Work out the finished part from the listing and answer in its coordinate system (mm). A direction names the side the tool comes from. Give positions to 0.01 mm unless a question says otherwise; leave off trailing zeros. Loops run counter-clockwise (first coordinate to the right, second up) from the corner with the lowest first, then second, coordinate; pieces in that order, holes last.
Autodesk Fusion 360 part; units mm, degrees
sketch "Sketch1" plane through (0, 0, 0) normal (0, 1, 0) x (1, 0, 0)
  circle A0 centre (0, 0) radius 4
  circle A1 centre (0, 0) radius 25
  line L0 (0, 0) -> (-25, 0)
  line L1 (0, 0) -> (25, 0)
  line L2 (-25, 0) -> (25, 0)
  line L3 (25, 0) -> (25, 51.781)
  line L4 (25, 51.781) -> (-25, 51.781)
  line L5 (-25, 51.781) -> (-25, 0)
  line L6 (-14.5, 51.781) -> (-7.5, 51.781)
  line L7 (-7.5, 51.781) -> (-7.5, 26.781)
  line L8 (-7.5, 26.781) -> (-14.5, 26.781)
  line L9 (-14.5, 26.781) -> (-14.5, 51.781)
  line L10 (-17.5, 35.781) -> (-4.5, 35.781)
  line L11 (-4.5, 35.781) -> (-4.5, 42.781)
  line L12 (-4.5, 42.781) -> (-17.5, 42.781)
  line L13 (-17.5, 42.781) -> (-17.5, 35.781)
  line L14 (-11, 35.781) -> (-11, 26.781)
  line L15 (-17.5, 39.281) -> (-14.5, 39.281)
  line L16 (0, 51.781) -> (0, 83.1045)
  line L17 (7.5, 51.781) -> (7.5, 26.781)
  line L18 (7.5, 26.781) -> (14.5, 26.781)
  line L19 (14.5, 26.781) -> (14.5, 51.781)
  line L20 (17.5, 35.781) -> (4.5, 35.781)
  line L21 (17.5, 42.781) -> (17.5, 35.781)
  line L22 (4.5, 42.781) -> (17.5, 42.781)
  line L23 (4.5, 35.781) -> (4.5, 42.781)
  dimension "d1" = 8
  dimension "d2" = 50
  dimension "d3" = 25
  dimension "d4" = 7
  dimension "d5" = 7
  dimension "d6" = 13
  dimension "d7" = 90
  dimension "d8" = 90
  dimension "d9" = 9
  dimension "d10" = 51.781
extrude "Extrude1" add sketch "Sketch1" along normal blind 10 contours A0 A1 L0 L1 L2 | A0 A1 L0 L1 L2 | A1 L3 L4 L5 L7 L8 L9 L10 L11 L12 L13 L17 L18 L19 L20 L21 L22 L23
extrude "Extrude2" add 1 faces at (14.2683, 0, -9.6781) along direction (0, -1, 0) blind 1
Item 1: Find section D-D, the plane z = 2. Write down the section's boundary in (x, y).
Item 2: Find section B-B, the plane z = -41. Write down the section's boundary in (x, y), plus the area to 3 significant figures.
Item 3: Consider line 1 (X direction, y = 8.25, z = -42); line 2 (X direction, y = 3, z = 0); line 3 (Z direction, x = 0, y = 7.25). Determine where each line is inside the solid, lowest interval first.
Item 4: For faces 5 (the face through (25, 5, -26)), 6 (the face through (-4.5, 5, -39)), 7 (the face through (7.5, 5, -47)), determine the directions among +Z, -Z, +X, -X, +Y, -Y from which every point of the face is accessible in a straight line to the end or side of a thin tool.
Item 5: Find section A-A, the plane x = 0. Write down the section's boundary in (y, z), plus the area to 3 significant figures.
Item 6: Determine the mould class of faces 1 (the face through (14.5, 5, -47)), 2 (the face through (-6, 5, -35.781)), 3 (the face through (-20, 5, -51.781)), 4 (the face through (-16, 5, -35.781)) for opening direction Z: released by +Z, released by -Z, zero draft, split by the parting line, or undercut.
Item 7: Flat-ended cylindrical pins translate along their axes: pin 1 Ø6.5 at (x, z) = (0, 0) entering from +Y; pin 2 Ø3 at (x, y) = (15.5, 9) entering from +Z; pin 3 Ø1 at (x, y) = (-16.5, 8) entering from +Z; pin 4 Ø2.5 at (x, y) = (-16, 2.5) entering from +Z. Find the tip coordinate at first contact, or state that the pin passes through.
Ans:
1. outline: (-24.92, -1) - (-3.46, -1) - (-3.46, 10) - (-24.92, 10) - close; (3.46, -1) - (24.92, -1) - (24.92, 10) - (3.46, 10) - close
2. outline: (-25, -1) - (-17.5, -1) - (-17.5, 10) - (-25, 10) - close; (-4.5, -1) - (4.5, -1) - (4.5, 10) - (-4.5, 10) - close; (17.5, -1) - (25, -1) - (25, 10) - (17.5, 10) - close
2. area: 264 mm2
3. line 1: x = -25 to -17.5, -4.5 to 4.5, 17.5 to 25
3. line 2: x = -25 to -4, 4 to 25
3. line 3: z = -51.78 to -4, 4 to 25
4. face 5: +Z, -Z, +X, +Y, -Y
4. face 6: +Y, -Y
4. face 7: -Z, +Y, -Y
5. outline: (-1, -51.78) - (10, -51.78) - (10, -4) - (-1, -4) - close; (-1, 4) - (10, 4) - (10, 25) - (-1, 25) - close
5. area: 757 mm2
6. face 1: zero draft
6. face 2: undercut
6. face 3: released by -Z
6. face 4: undercut
7. pin 1: passes through
7. pin 2: stops at z = 20.71
7. pin 3: stops at z = 19.21
7. pin 4: stops at z = 20.19
